For this review, use the dimensioned drawing (mm, ordinates from the lowest corner) and the shaded views. A direction names the side the tool comes from. Give positions to 0.01 mm unless a question says otherwise; leave off trailing zeros. Loops run counter-clockwise (first coordinate to the right, second up) from the corner with the lowest first, then second, coordinate; pieces in that order, holes last. Notation, with made-up numbers: (14.5, 79) - (60.5, 79) arc R12 cw to (60.5, 96) - close; hole circle Ø10 at (60, 68). An arc over 180 degrees is marked (long way). Write each question's results on one line, items separated by ' | '.
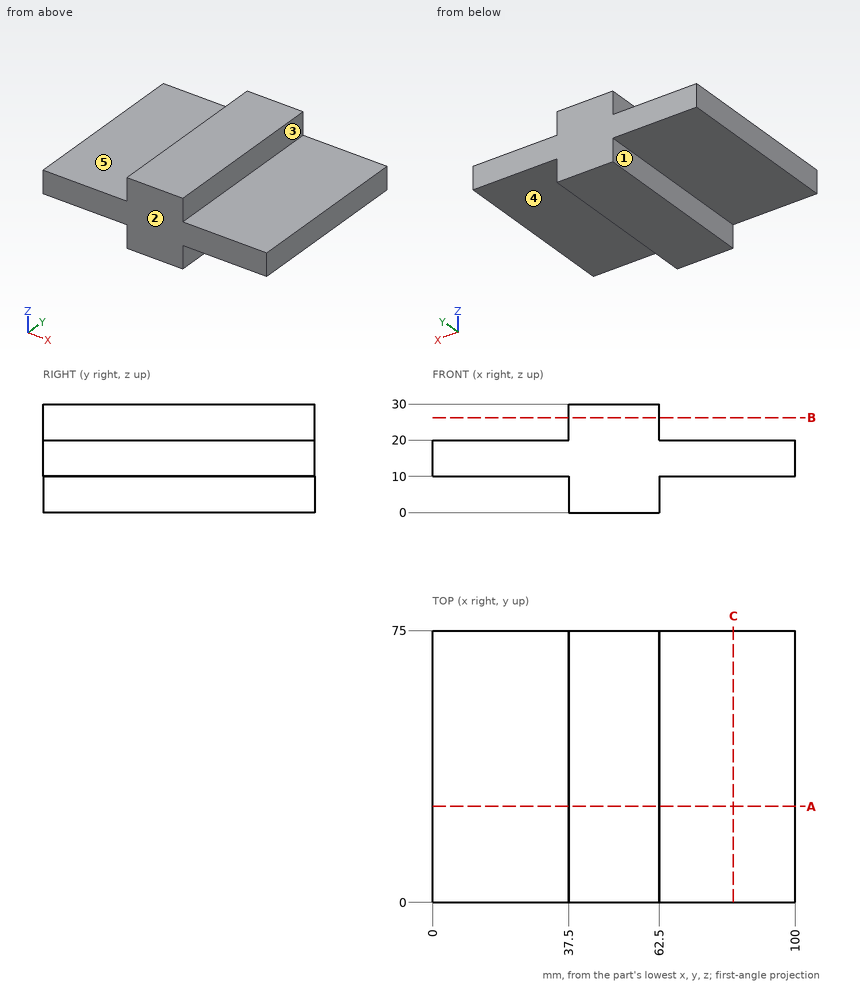
Item 1: Clearance check with flat-ended pins moving along their axes: P1, Ø3, axis at x = 32.5, y = 53.5, coming from the +Z side; P2, Ø11, axis at x = 72.5, y = 21, coming from the -Z side. State where each tip first meets the part, or that it passes through.
Output values:
P1: stops at z = 20 | P2: stops at z = 10
Item 2: We need section C-C on x = 83. Give the boundary of the cut face in (y, z), then the cut area to 3 significant figures.
Output values:
outline: (0, 10) - (75, 10) - (75, 20) - (0, 20) - close | area: 750 mm²
Item 3: Wall thickness on probe 1 along X at (y, z) = (68.5, 9.75); probe 2 along Z at (x, y) = (86, 32.5): over which ranges is each line inside the solid? List them lowest first.
Output values:
probe 1: x = 37.5 to 62.5 | probe 2: z = 10 to 20
Item 4: We need section B-B on z = 26.25. Give the boundary of the cut face in (x, y).
Output values:
outline: (37.5, 0) - (62.5, 0) - (62.5, 75) - (37.5, 75) - close
Item 5: Tool access review of the marked faces 1, 2, 3, 4 and 5: name each direction out of +Z, -Z, +X, -X, +Y, -Y from which nothing blocks a thin tool from reaching the whole face with its end or side.
Output values:
face 1: -Z, -X, +Y, -Y | face 2: +Z, -Z, +X, -X, -Y | face 3: +Z, +X, +Y, -Y | face 4: -Z, +X, +Y, -Y | face 5: +Z, -X, +Y, -Y
Item 6: We need section A-A on y = 26.5. Give the boundary of the cut face in (x, z), then the cut area to 3 significant figures.
Output values:
outline: (0, 10) - (37.5, 10) - (37.5, 0) - (62.5, 0) - (62.5, 10) - (100, 10) - (100, 20) - (62.5, 20) - (62.5, 30) - (37.5, 30) - (37.5, 20) - (0, 20) - close | area: 1,500 mm²
